```python
from build123d import *

# Parameters (mm, degrees)
F1_DEPTH = 1.5
F2_W     = 19
F2_H     = 23
F3_DEPTH = 1.2
F4_R     = 2


with BuildPart() as f1:
    # F0 (on Top) → F1 (new body)
    with BuildSketch(Plane.XY):
        Polygon((33.25, -61.25), (33.25, 61.25), (0, 61.25), (-33.25, 61.25), (-33.25, -61.25), (0, -61.25), align=None)
        Polygon((24.75, -58.25), (0, -58.25), (-24.75, -58.25), (-24.75, -41.75), (-8.25, -41.75), (-8.25, -25.25), (8.25, -25.25), (8.25, -41.75), (24.75, -41.75), align=None, mode=Mode.SUBTRACT)
        Polygon((-24.75, 35.25), (0, 35.25), (24.75, 35.25), (24.75, 2.25), (-24.75, 2.25), align=None, mode=Mode.SUBTRACT)
        Polygon((-24.75, 58.25), (0, 58.25), (24.75, 58.25), (24.75, 41.75), (0, 41.75), (-24.75, 41.75), align=None, mode=Mode.SUBTRACT)
    extrude(amount=F1_DEPTH)

    # F2 (on face) → F3 (cut)
    with BuildSketch(Plane(origin=(0, 0, 0), x_dir=(1, 0, 0), z_dir=(0, 0, -1))):
        with Locations((9.5, 11.5)):
            Rectangle(F2_W, F2_H)
        with Locations((-9.5, 11.5)):
            Rectangle(F2_W, F2_H)
    extrude(amount=-F3_DEPTH, mode=Mode.SUBTRACT)

    # F4
    f4_edges = [f1.edges().sort_by_distance(p)[0] for p in [
        (33.25, -61.25, 0.75),
        (33.25, 61.25, 0.75),
    ]]
    fillet(f4_edges, radius=F4_R)


solid = f1.part
```
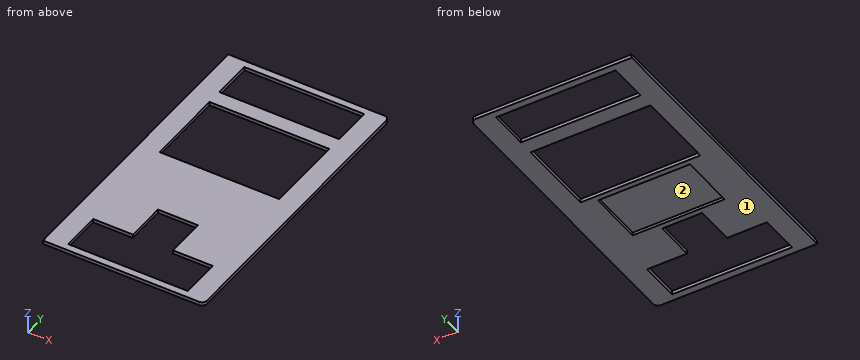
Here's how the part is built. I have some questions about the finished solid (model axes, mm). Face numbers are marked on the shaded views. Coordinates: 2 decimals unless noted, no trailing zeros. Loops run counter-clockwise (first coordinate to the right, second up) from the corner with the lowest first, then second, coordinate; pieces in that order, holes last. Notation, with made-up numbers: (35, -38.5) - (46, -38.5) arc R24 cw to (46, -22.5) - close; hole circle Ø10 at (-10, 50). An arc over 180 degrees is marked (long way). Return JSON: item names as keys, results as strings. Group by question number.
Item 1: If we section it at D-D on y = -2: Write out the boundary of the cut face in (x, z).
Item 2: If we section it at C-C on z = 0.85: Write out the boundary of the cut face in (x, y).
Item 3: If we section it at A-A on x = 10.5: Write out the boundary of the cut face in (y, z).
Item 4: Will this pin go through, and if not, where does the flat tip stop? P1, Ø11.5, axis at x = -7, y = -13.5, coming from the -Z side.
Item 5: We'd pull the mould along X, two halves only. Please class the marked faces 1 and 2: +X half, -X half, draft (parallel to the pull), parting line (faces both ways), or undercut.
Item 6: If we section it at B-B on y = 15.5: Write out the boundary of the cut face in (x, z).
Item 7: I need wall thicknesses on line 1 (Y direction, x = 7.5, z = 1.1); line 2 (Y direction, x = -21, z = 0.3); line 3 (Y direction, x = -9, z = 0.3). Which ranges of each line are inside material? Lowest first, please. Write a range as from..to.
Calculated:
{
 "1": {"outline": "(-33.25, 0) - (-19, 0) - (-19, 1.2) - (19, 1.2) - (19, 0) - (33.25, 0) - (33.25, 1.5) - (-33.25, 1.5) - close"},
 "2": {"outline": "(-33.25, -61.25) - (31.25, -61.25) arc R2 ccw to (33.25, -59.25) - (33.25, 59.25) arc R2 ccw to (31.25, 61.25) - (-33.25, 61.25) - close; hole (-24.75, -58.25) - (24.75, -58.25) - (24.75, -41.75) - (8.25, -41.75) - (8.25, -25.25) - (-8.25, -25.25) - (-8.25, -41.75) - (-24.75, -41.75) - close; hole (-24.75, 2.25) - (24.75, 2.25) - (24.75, 35.25) - (-24.75, 35.25) - close; hole (-24.75, 41.75) - (24.75, 41.75) - (24.75, 58.25) - (-24.75, 58.25) - close; hole (-19, -23) - (19, -23) - (19, 0) - (-19, 0) - close"},
 "3": {"outline": "(-61.25, 0) - (-58.25, 0) - (-58.25, 1.5) - (-61.25, 1.5) - close; (-41.75, 0) - (-23, 0) - (-23, 1.2) - (0, 1.2) - (0, 0) - (2.25, 0) - (2.25, 1.5) - (-41.75, 1.5) - close; (35.25, 0) - (41.75, 0) - (41.75, 1.5) - (35.25, 1.5) - close; (58.25, 0) - (61.25, 0) - (61.25, 1.5) - (58.25, 1.5) - close"},
 "4": {"P1": "stops at z = 1.2"},
 "5": {"face 1": "draft", "face 2": "undercut"},
 "6": {"outline": "(-33.25, 0) - (-24.75, 0) - (-24.75, 1.5) - (-33.25, 1.5) - close; (24.75, 0) - (33.25, 0) - (33.25, 1.5) - (24.75, 1.5) - close"},
 "7": {"line 1": "y = -61.25..-58.25, -25.25..-23, 0..2.25, 35.25..41.75, 58.25..61.25", "line 2": "y = -61.25..-58.25, -41.75..2.25, 35.25..41.75, 58.25..61.25", "line 3": "y = -61.25..-58.25, -41.75..-23, 0..2.25, 35.25..41.75, 58.25..61.25"}
}
